Answer from the drawing. Dimensions are ordinates in mm from the lowest x, y and z of the part. A direction names the side the tool comes from. Coordinates: 2 decimals unless noted, no trailing zeros. Write each loop counter-clockwise with the first axis right and the second up, starting at its lowest first coordinate (ties: lowest second). Pieces come first, ordered by that corner, then holes. Notation, with made-up numbers: (66.5, -13.5) -> (95.5, -13.5) arc R26 ccw to (95.5, 0.5) -> close; hole circle Ø3 at (28, 11.25). An arc over 180 degrees is marked (long way). One line per item, written item: value. Start each with the question number.
1. Find section B-B, the plane z = 3.25. Write down the section's boundary in (x, y).
2. Find section D-D, the plane x = 14.5. Write down the section's boundary in (y, z), and give its area (3 significant figures).
3. Given P1, Ø1, axis at x = 36.5, z = 2, coming from the +Y side; P2, Ø4, axis at x = 16, y = 19, coming from the -Z side; P3, Ø5, axis at x = 17.5, y = 8.5, coming from the +Z side; P4, Ø4, axis at y = 22, z = 2.5, coming from the -X side (1 decimal), each flat-ended and moving along its own axis, determine where each tip first touches the part or whether it passes through.
4. For the marked faces 1 and 2, determine the directions among +Z, -Z, +X, -X, +Y, -Y from which every point of the face is accessible in a straight line to the end or side of a thin tool.
5. Find section C-C, the plane y = 7.75. Write down the section's boundary in (x, z).
6. Consider line 1 along Z through (x, y) = (19.5, 22.5); line 2 along Z through (x, y) = (36, 12.5); line 3 along Y through (x, z) = (42.25, 2.9) (1 decimal). Determine where each line is inside the solid, lowest interval first.
7. For a pull along X with two mould halves and no side action, classify the marked faces 3, 4 and 5 as pulls with the +X half, pulls with the -X half, needs draft (parallel to the pull), parting line crosses it, or undercut.
8. Find section A-A, the plane x = 24. Write down the section's boundary in (y, z), and give its area (3 significant figures).
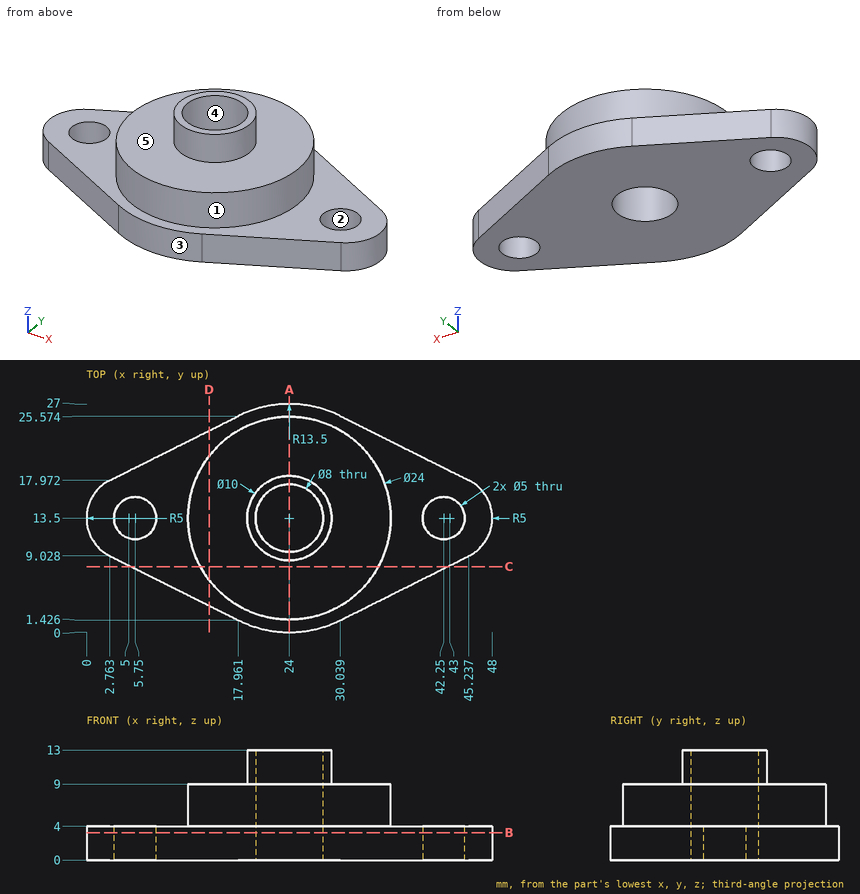
Answer block:
1. outline: (2.76, 9.03) -> (17.96, 1.43) arc R13.5 ccw to (30.04, 1.43) -> (45.24, 9.03) arc R5 ccw to (45.24, 17.97) -> (30.04, 25.57) arc R13.5 ccw to (17.96, 25.57) -> (2.76, 17.97) arc R5 ccw to start; hole circle Ø5 at (5.75, 13.5); hole circle Ø8 at (24, 13.5); hole circle Ø5 at (42.25, 13.5)
2. outline: (3.16, 0) -> (23.84, 0) -> (23.84, 4) -> (20.83, 4) -> (20.83, 9) -> (6.17, 9) -> (6.17, 4) -> (3.16, 4) -> close
2. area: 156 mm2
3. P1: stops at y = 22.59
3. P2: stops at z = 0
3. P3: stops at z = 9
3. P4: stops at x = 6.8
4. face 1: +Z
4. face 2: +Z, -Z
5. outline: (5.32, 0) -> (42.68, 0) -> (42.68, 4) -> (34.53, 4) -> (34.53, 9) -> (13.47, 9) -> (13.47, 4) -> (5.32, 4) -> close
6. line 1: z = 0 to 9
6. line 2: z = 0 to 4
6. line 3: y = 7.5 to 11, 16 to 19.5
7. face 3: parting line crosses it
7. face 4: undercut
7. face 5: needs draft
8. outline: (0, 0) -> (9.5, 0) -> (9.5, 13) -> (8.5, 13) -> (8.5, 9) -> (1.5, 9) -> (1.5, 4) -> (0, 4) -> close; (17.5, 0) -> (27, 0) -> (27, 4) -> (25.5, 4) -> (25.5, 9) -> (18.5, 9) -> (18.5, 13) -> (17.5, 13) -> close
8. area: 164 mm2
